Check sheet for the modelled part. Datum: model origin and axes. Units: mm. A direction names the side the tool comes from. Coordinates: 2 decimals unless noted, no trailing zeros. Loops run counter-clockwise (first coordinate to the right, second up) from the corner with the lowest first, then second, coordinate; pieces in that order, holes last.
Autodesk Inventor part; units mm, degrees
ref_plane "YZ Plane" through (0, 0, 0) normal (1, 0, 0) x (0, 1, 0)
ref_plane "XZ Plane" through (0, 0, 0) normal (0, 1, 0) x (-1, 0, 0)
ref_plane "XY Plane" through (0, 0, 0) normal (0, 0, 1) x (1, 0, 0)
sketch "Boceto1" plane through (0, 0, 0) normal (0, 0, 1) x (1, 0, 0)
  line L0 (-35, 0) -> (15, 0)
  line L1 (-20, 10) -> (-20, 0)
  arc A0 (-10, 20) -> (-20, 10) centre (-10, 10) ccw
  arc A1 (-10, 25) -> (-25, 10) centre (-10, 10) ccw
  line L2 (-25, 10) -> (-25, 0)
  arc A2 (-10, 35) -> (-35, 10) centre (-10, 10) ccw
  line L3 (-35, 10) -> (-35, 0)
  line L4 (-35, 0) -> (-10, 0)
  circle A3 centre (-10, 10) radius 2.5
  line L5 (-10, 20) -> (0, 20)
  line L6 (0, 20) -> (0, 21.1803)
  line L7 (0, 25) -> (-10, 25)
  line L8 (-10, 35) -> (0, 35)
  line L9 (0, 35) -> (0, 25)
  line L10 (0, 20) -> (0, 0)
  line L11 (0, 0) -> (-10, 0)
  line L12 (0, 25) -> (0, 20)
  line L13 (-10, 25) -> (-10, 20)
  line L14 (-20, 5) -> (-25, 5)
  point P0 (0, 0)
  dimension "d0" = 20
  dimension "d1" = 25
  dimension "d2" = 10
  dimension "d3" = 10
  dimension "d4" = 5
  dimension "d6" = 35
extrude "Extrusión1" add sketch "Boceto1" along normal mid plane 5 contours L3 A2 L8 L9 L7 A1 L2 L0 | L2 L14 L1 L0 | L1 A0 L5 L10 L0 | L7 L12 L6 L5 L13
sketch "Boceto2" plane through (0, 0, 2.5) normal (0, 0, 1) x (1, 0, 0)
  circle A0 centre (-10, 10) radius 2.3
  circle A1 centre (-22.5, 10) radius 2.3
  circle A2 centre (-10, 10) radius 2.5
  point P0 (0, 0)
  dimension "d9" = 4.6
  dimension "d10" = 4.6
extrude "Extrusión2" add sketch "Boceto2" along normal blind 0.4 and the other way blind 5.4 contours A0 | A1
sketch "Boceto3" plane through (-10, 10, 2.9) normal (0, 0, 1) x (1, 0, 0)
  arc A0 (5, 0) -> (0.4927, 4.9757) centre (0, 0) ccw
  line L0 (-30, 0) -> (-30, 7.9951)
  line L1 (0.4927, 4.9757) -> (-30, 7.9951)
  line L2 (-30, 0) -> (-30, -7.9951)
  line L3 (0.4927, -4.9757) -> (-30, -7.9951)
  arc A1 (0.4927, -4.9757) -> (5, 0) centre (0, 0) ccw
  circle A2 centre (0, 0) radius 2.3
  point P0 (10, -10)
  dimension "d15" = 10
extrude "Extrusión3" add sketch "Boceto3" along normal blind 5 contours A1 L3 L2 L0 L1 A0 | A2
sketch "Boceto4" plane through (-22.5, 10, -2.9) normal (0, 0, -1) x (-1, 0, 0)
  circle A0 centre (0, 0) radius 2.3
  circle A1 centre (-12.5, 0) radius 2.3
  line L0 (-12.9927, 4.9757) -> (17.5, 7.9951)
  arc A2 (-12.9927, 4.9757) -> (-12.9927, -4.9757) centre (-12.5, 0) ccw
  line L1 (17.5, -7.9951) -> (-12.9927, -4.9757)
  line L2 (17.5, 7.9951) -> (17.5, -7.9951)
  point P0 (-22.5, -10)
extrude "Extrusión4" add sketch "Boceto4" along normal blind 5 contours A0 | A1 | L0 L2 L1 A2
sketch "Boceto5" plane through (0, 0, -2.5) normal (0, 0, -1) x (-1, 0, 0)
  circle A0 centre (10, 10) radius 2.3
  circle A1 centre (10, 10) radius 0.4
  line L0 (10, 10) -> (10, 1.6419)
  line L1 (10, 1.6419) -> (12.8355, 1.6419)
  circle A2 centre (10, 6) radius 0.4
  circle A3 centre (10, 6) radius 0.4
  circle A4 centre (14, 10) radius 0.4
  circle A5 centre (14, 6) radius 0.4
  circle A6 centre (12, 6) radius 0.4
  circle A7 centre (18, 10) radius 0.4
  circle A8 centre (18, 6) radius 0.4
  circle A9 centre (14, 6) radius 0.4
  circle A10 centre (22, 10) radius 0.4
  circle A11 centre (22, 6) radius 0.4
  circle A12 centre (16, 6) radius 0.4
  circle A13 centre (26, 10) radius 0.4
  circle A14 centre (26, 6) radius 0.4
  circle A15 centre (18, 6) radius 0.4
  circle A16 centre (30, 10) radius 0.4
  circle A17 centre (30, 6) radius 0.4
  circle A18 centre (20, 6) radius 0.4
  circle A19 centre (34, 10) radius 0.4
  circle A20 centre (34, 6) radius 0.4
  circle A21 centre (22, 6) radius 0.4
  circle A22 centre (24, 10) radius 0.4
  circle A23 centre (24, 8) radius 0.4
  circle A24 centre (24, 6) radius 0.4
  circle A25 centre (26, 10) radius 0.4
  circle A26 centre (26, 8) radius 0.4
  circle A27 centre (26, 6) radius 0.4
  circle A28 centre (28, 10) radius 0.4
  circle A29 centre (28, 8) radius 0.4
  circle A30 centre (28, 6) radius 0.4
  circle A31 centre (30, 10) radius 0.4
  circle A32 centre (30, 8) radius 0.4
  circle A33 centre (30, 6) radius 0.4
  circle A34 centre (32, 10) radius 0.4
  circle A35 centre (32, 8) radius 0.4
  circle A36 centre (32, 6) radius 0.4
  circle A37 centre (34, 10) radius 0.4
  circle A38 centre (34, 8) radius 0.4
  circle A39 centre (34, 6) radius 0.4
  circle A40 centre (36, 10) radius 0.4
  circle A41 centre (36, 8) radius 0.4
  circle A42 centre (36, 6) radius 0.4
  circle A43 centre (38, 10) radius 0.4
  circle A44 centre (38, 8) radius 0.4
  circle A45 centre (38, 6) radius 0.4
  circle A46 centre (10, 14) radius 0.4
  line L2 (10, 14) -> (10, 5.6419)
  circle A47 centre (10, 10) radius 0.4
  circle A48 centre (18, 14) radius 0.4
  circle A49 centre (18, 10) radius 0.4
  circle A50 centre (14, 10) radius 0.4
  circle A51 centre (14, 14) radius 0.4
  circle A52 centre (14, 10) radius 0.4
  circle A53 centre (12, 10) radius 0.4
  circle A54 centre (10, 10) radius 0.4
  circle A55 centre (16, 10) radius 0.4
  circle A56 centre (34, 14) radius 0.4
  circle A57 centre (34, 10) radius 0.4
  circle A58 centre (22, 10) radius 0.4
  circle A59 centre (24, 10) radius 0.4
  circle A60 centre (24, 12) radius 0.4
  circle A61 centre (24, 14) radius 0.4
  circle A62 centre (26, 10) radius 0.4
  circle A63 centre (26, 14) radius 0.4
  circle A64 centre (26, 12) radius 0.4
  circle A65 centre (28, 14) radius 0.4
  circle A66 centre (28, 12) radius 0.4
  circle A67 centre (28, 10) radius 0.4
  circle A68 centre (30, 10) radius 0.4
  circle A69 centre (30, 12) radius 0.4
  circle A70 centre (30, 14) radius 0.4
  circle A71 centre (32, 10) radius 0.4
  circle A72 centre (32, 12) radius 0.4
  circle A73 centre (32, 14) radius 0.4
  circle A74 centre (34, 14) radius 0.4
  circle A75 centre (34, 12) radius 0.4
  circle A76 centre (34, 10) radius 0.4
  circle A77 centre (36, 12) radius 0.4
  circle A78 centre (36, 10) radius 0.4
  circle A79 centre (36, 14) radius 0.4
  circle A80 centre (38, 10) radius 0.4
  circle A81 centre (38, 12) radius 0.4
  circle A82 centre (38, 14) radius 0.4
  circle A83 centre (22, 10) radius 0.4
  circle A84 centre (26, 10) radius 0.4
  circle A85 centre (18, 10) radius 0.4
  circle A86 centre (26, 14) radius 0.4
  circle A87 centre (20, 10) radius 0.4
  circle A88 centre (30, 10) radius 0.4
  circle A89 centre (30, 14) radius 0.4
  circle A90 centre (22, 14) radius 0.4
  circle A91 centre (12, 10) radius 0.4
  circle A92 centre (12, 6) radius 0.4
  circle A93 centre (8, 6) radius 0.4
  circle A94 centre (8, 10) radius 0.4
  circle A95 centre (8, 6) radius 0.4
  circle A96 centre (6, 6) radius 0.4
  circle A97 centre (12, 14) radius 0.4
  circle A98 centre (12, 10) radius 0.4
  circle A99 centre (8, 10) radius 0.4
  circle A100 centre (8, 14) radius 0.4
  circle A101 centre (8, 10) radius 0.4
  circle A102 centre (6, 10) radius 0.4
  point P0 (0, 0)
  dimension "d20" = 0.8
  dimension "d23" = 4
  dimension "d26" = 4
  dimension "d31" = 4
  dimension "d38" = 6
extrude "Extrusión5" add sketch "Boceto5" along normal up to next contours A2 L0 | L0 A2 | A46 | A4 | A5 | A7 | A8 | A13 | A14 | A16 | A17 | A19 | A20 | A48 | A51 | A56 | A63 | A70 | A102
mirror "Simetría1" about plane through (0, 0, 0) normal (0, 0, 1) of "Extrusión5"
properties part number "Prueba de soportes mecanismo_3DPrint"
(1) Section check C-C, the plane x = -17. Enter the section's corners in (y, z), plus the area to 3 significant figures.
(2) Draft check along X on faces 5 (the face through (-10, 23, 0)), 6 (the face through (-6, 13, 5)), 7 (the face through (-40, 10, -5)). Enter one of: pulls with the +X half, pulls with the -X half, needs draft (parallel to the pull), parting line crosses it, or undercut.
(3) Section check A-A, the plane z = 1. Enter the section's corners in (x, y).
(4) Section check B-B, the plane x = -31. Enter the section's corners in (y, z), plus the area to 3 significant figures.
(5) Scan lines: line 1 along Z through (x, y) = (-30.5, 13); line 2 along Y through (x, z) = (-22, 0.75) (3 decimals); line 3 along Z through (x, y) = (-22, 13). Record each from-to range of solid material in increasing order.
(6) Set-up check for faces 1 (the face through (-25, 8, 0)), 2 (the face through (-6, 7, 5)), 3 (the face through (-24.967, 3.493, -5.365)), 4 (the face through (-27.871, 27.482, -0.035)): record each of +Z, -Z, +X, -X, +Y, -Y from which the full face is reachable in a straight line by a thin tool's end or side.
(7) Section check D-D, the plane x = -22.5. Enter the section's corners in (y, z), plus the area to 3 significant figures.
(8) Gauge pin test, flat ends, axial feed: P1, Ø2, axis at x = -13.5, y = 27, coming from the +Z side; P2, Ø4, axis at x = -25, y = 26.5, coming from the -Z side; P3, Ø1.5, axis at x = -22, z = -0.5, coming from the +Y side; P4, Ø1, axis at x = -33.5, y = 22, coming from the -Z side. Record the tip position at first contact, or that the pin passes through.
Determined:
1. outline: (0, -2.5) - (17.14, -2.5) - (17.14, 2.5) - (0, 2.5) - close; (4.28, -7.9) - (15.72, -7.9) - (15.72, -2.9) - (4.28, -2.9) - close; (4.28, 2.9) - (15.72, 2.9) - (15.72, 7.9) - (4.28, 7.9) - close; (23.27, -2.5) - (34, -2.5) - (34, 2.5) - (23.27, 2.5) - close
1. area: 254 mm2
2. face 5: undercut
2. face 6: pulls with the +X half
2. face 7: pulls with the -X half
3. outline: (-35, 0) - (0, 0) - (0, 35) - (-10, 35) arc R25 ccw to (-35, 10) - close; circle Ø4.6 at (-22.5, 10); circle Ø4.6 at (-10, 10); hole (-25, 5) - (-20, 5) - (-20, 10) arc R10 cw to (-10, 20) - (-10, 25) arc R15 ccw to (-25, 10) - close; hole circle Ø5 at (-10, 10)
4. outline: (0, -2.5) - (23.56, -2.5) - (23.56, 2.5) - (0, 2.5) - close; (2.9, -7.9) - (17.1, -7.9) - (17.1, -2.9) - (2.9, -2.9) - close; (2.9, 2.9) - (17.1, 2.9) - (17.1, 7.9) - (2.9, 7.9) - close
4. area: 260 mm2
5. line 1: z = -7.9 to -2.9, -2.5 to 2.5, 2.9 to 7.9
5. line 2: y = 0 to 5, 7.755 to 12.245, 19 to 31.932
5. line 3: z = -7.9 to -2.9, 2.9 to 7.9
6. face 1: none
6. face 2: +Z, +X, -Y
6. face 3: -Z, +X, -Y
6. face 4: -X, +Y
7. outline: (0, -2.5) - (5, -2.5) - (5, 2.5) - (0, 2.5) - close; (3.74, -7.9) - (16.26, -7.9) - (16.26, -2.9) - (12.3, -2.9) - (12.3, 2.9) - (16.26, 2.9) - (16.26, 7.9) - (3.74, 7.9) - (3.74, 2.9) - (7.7, 2.9) - (7.7, -2.9) - (3.74, -2.9) - close; (18.29, -2.5) - (31.65, -2.5) - (31.65, 2.5) - (18.29, 2.5) - close
7. area: 244 mm2
8. P1: stops at z = 2.5
8. P2: stops at z = -2.5
8. P3: stops at y = 32.33
8. P4: passes through
